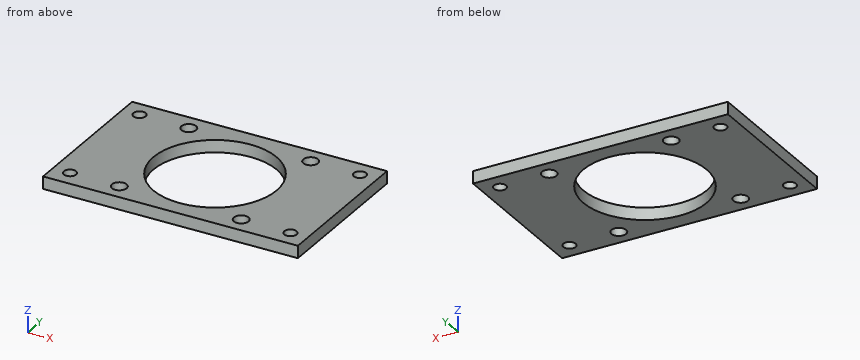
```python
from build123d import *

# Parameters (mm, degrees)
SKETCH1_W           = 103.497474684
SKETCH1_H           = 63.497474684
SKETCH1_R           = 25
SKETCH1_R_2         = 3
SKETCH1_R_3         = 2.5
BOSS_EXTRUDE1_DEPTH = 5


with BuildPart() as part:
    # Sketch1 → Boss-Extrude1 (new body)
    with BuildSketch(Plane.XY):
        Rectangle(SKETCH1_W, SKETCH1_H)
        Circle(SKETCH1_R, mode=Mode.SUBTRACT)
        with Locations((24.748737342, 24.748737342)):
            Circle(SKETCH1_R_2, mode=Mode.SUBTRACT)
        with Locations((24.748737342, -24.748737342)):
            Circle(SKETCH1_R_2, mode=Mode.SUBTRACT)
        with Locations((-24.748737342, -24.748737342)):
            Circle(SKETCH1_R_2, mode=Mode.SUBTRACT)
        with Locations((-24.748737342, 24.748737342)):
            Circle(SKETCH1_R_2, mode=Mode.SUBTRACT)
        with Locations((44.748737342, 24.748737342)):
            Circle(SKETCH1_R_3, mode=Mode.SUBTRACT)
        with Locations(Location((44.748737342, -24.748737342, 0), (0, 0, 180))):
            Circle(SKETCH1_R_3, mode=Mode.SUBTRACT)
        with Locations((-44.748737342, -24.748737342)):
            Circle(SKETCH1_R_3, mode=Mode.SUBTRACT)
        with Locations(Location((-44.748737342, 24.748737342, 0), (0, 0, 180))):
            Circle(SKETCH1_R_3, mode=Mode.SUBTRACT)
    extrude(amount=BOSS_EXTRUDE1_DEPTH)


solid = part.part
```
Input: part model. Units: mm. Frame: model coordinates. Give positions to 0.01 mm unless a question says otherwise; leave off trailing zeros. Order: outer loops, then holes, each group sorted by start corner. A loop starts at its lowest first (then second) coordinate and runs counter-clockwise, first axis right, second up.
1. Line query: probe 1 along Y at (x, z) = (0, 2.75); probe 2 along Y at (x, z) = (-43.5, 3.2); probe 3 along Y at (x, z) = (22.5, 2.1). Output: solid intervals per line, ascending.
Computed:
probe 1: y = -31.75 to -25, 25 to 31.75
probe 2: y = -31.75 to -26.91, -22.58 to 22.58, 26.91 to 31.75
probe 3: y = -31.75 to -26.73, -22.76 to -10.9, 10.9 to 22.76, 26.73 to 31.75
2. Cut plane A-A (x = 0). Return loops of the section in (y, z), and give its area (3 significant figures).
Computed:
outline: (-31.75, 0) - (-25, 0) - (-25, 5) - (-31.75, 5) - close; (25, 0) - (31.75, 0) - (31.75, 5) - (25, 5) - close
area: 67.5 mm2
3. Cut plane C-C (z = 0.9). State how many separate pieces and enclosed holes the cut face has, and give its area (3 significant figures).
Computed:
separate pieces: 1
enclosed holes: 9
area: 4,420 mm2
4. Cut plane B-B (y = 0). Return loops of the section in (x, z), and give its area (3 significant figures).
Computed:
outline: (-51.75, 0) - (-25, 0) - (-25, 5) - (-51.75, 5) - close; (25, 0) - (51.75, 0) - (51.75, 5) - (25, 5) - close
area: 267 mm2
